```python
from build123d import *

# Parameters (mm, degrees)
F0_W     = 69.5
F0_H     = 23
F0_R     = 5.75
F0_W_2   = 1
F0_H_2   = 4
F1_DEPTH = 2
F0_R_2   = 5.25
F2_DEPTH = 10


with BuildPart() as f1:
    # F0 (on Top) → F1 (new body)
    with BuildSketch(Plane.XY):
        with Locations((3.4471642077, -3.0003356891)):
            Rectangle(F0_W, F0_H)
        Polygon((-29.8028357923, -13.0003356891), (-29.8028357923, 6.9996643109), (-15.8028357923, 6.9996643109), (-14.8028357923, 6.9996643109), (-13.3028357923, 6.9996643109), (-12.3028357923, 6.9996643109), (1.6971642077, 6.9996643109), (2.6971642077, 6.9996643109), (4.1971642077, 6.9996643109), (5.1971642077, 6.9996643109), (19.1971642077, 6.9996643109), (20.1971642077, 6.9996643109), (21.6971642077, 6.9996643109), (22.6971642077, 6.9996643109), (36.6971642077, 6.9996643109), (36.6971642077, -13.0003356891), (22.6971642077, -13.0003356891), (21.6971642077, -13.0003356891), (20.1971642077, -13.0003356891), (19.1971642077, -13.0003356891), (5.1971642077, -13.0003356891), (5.1971642077, -9.0003356891), (4.1971642077, -9.0003356891), (4.1971642077, -13.0003356891), (2.6971642077, -13.0003356891), (1.6971642077, -13.0003356891), (-12.3028357923, -13.0003356891), (-13.3028357923, -13.0003356891), (-14.8028357923, -13.0003356891), (-15.8028357923, -13.0003356891), align=None, mode=Mode.SUBTRACT)
        Polygon((-15.8028357923, 6.9996643109), (-29.8028357923, 6.9996643109), (-29.8028357923, -13.0003356891), (-15.8028357923, -13.0003356891), (-15.8028357923, -9.0003356891), (-14.8028357923, -9.0003356891), (-14.8028357923, -13.0003356891), (-13.3028357923, -13.0003356891), (-13.3028357923, -9.0003356891), (-12.3028357923, -9.0003356891), (-12.3028357923, -13.0003356891), (1.6971642077, -13.0003356891), (1.6971642077, -9.0003356891), (2.6971642077, -9.0003356891), (2.6971642077, -13.0003356891), (4.1971642077, -13.0003356891), (4.1971642077, -9.0003356891), (5.1971642077, -9.0003356891), (5.1971642077, -13.0003356891), (19.1971642077, -13.0003356891), (19.1971642077, -9.0003356891), (20.1971642077, -9.0003356891), (20.1971642077, -13.0003356891), (21.6971642077, -13.0003356891), (21.6971642077, -9.0003356891), (22.6971642077, -9.0003356891), (22.6971642077, -13.0003356891), (36.6971642077, -13.0003356891), (36.6971642077, 6.9996643109), (22.6971642077, 6.9996643109), (22.6971642077, 2.9996643109), (21.6971642077, 2.9996643109), (21.6971642077, 6.9996643109), (20.1971642077, 6.9996643109), (20.1971642077, 2.9996643109), (19.1971642077, 2.9996643109), (19.1971642077, 6.9996643109), (5.1971642077, 6.9996643109), (5.1971642077, 2.9996643109), (4.1971642077, 2.9996643109), (4.1971642077, 6.9996643109), (2.6971642077, 6.9996643109), (2.6971642077, 2.9996643109), (1.6971642077, 2.9996643109), (1.6971642077, 6.9996643109), (-12.3028357923, 6.9996643109), (-12.3028357923, 2.9996643109), (-13.3028357923, 2.9996643109), (-13.3028357923, 6.9996643109), (-14.8028357923, 6.9996643109), (-14.8028357923, 2.9996643109), (-15.8028357923, 2.9996643109), align=None)
        with Locations((-22.8028357923, -3.0003356891)):
            Circle(F0_R, mode=Mode.SUBTRACT)
        with Locations((-5.3028357923, -3.0003356891)):
            Circle(F0_R, mode=Mode.SUBTRACT)
        with Locations((12.1971642077, -3.0003356891)):
            Circle(F0_R, mode=Mode.SUBTRACT)
        with Locations((29.6971642077, -3.0003356891)):
            Circle(F0_R, mode=Mode.SUBTRACT)
        with Locations((-15.3028357923, 4.9996643109)):
            Rectangle(F0_W_2, F0_H_2)
        with Locations((-12.8028357923, 4.9996643109)):
            Rectangle(F0_W_2, F0_H_2)
        with Locations((2.1971642077, 4.9996643109)):
            Rectangle(F0_W_2, F0_H_2)
        with Locations((4.6971642077, 4.9996643109)):
            Rectangle(F0_W_2, F0_H_2)
        with Locations((19.6971642077, 4.9996643109)):
            Rectangle(F0_W_2, F0_H_2)
        with Locations((22.1971642077, 4.9996643109)):
            Rectangle(F0_W_2, F0_H_2)
        with Locations((-15.3028357923, -11.0003356891)):
            Rectangle(F0_W_2, F0_H_2)
        with Locations((-12.8028357923, -11.0003356891)):
            Rectangle(F0_W_2, F0_H_2)
        with Locations((2.1971642077, -11.0003356891)):
            Rectangle(F0_W_2, F0_H_2)
        with Locations((19.6971642077, -11.0003356891)):
            Rectangle(F0_W_2, F0_H_2)
        with Locations((22.1971642077, -11.0003356891)):
            Rectangle(F0_W_2, F0_H_2)
    extrude(amount=F1_DEPTH)

    # F0 (on Top) → F2 (join)
    with BuildSketch(Plane.XY):
        with Locations((-22.8028357923, -3.0003356891)):
            Circle(F0_R)
        with Locations((-22.8028357923, -3.0003356891)):
            Circle(F0_R_2, mode=Mode.SUBTRACT)
        with Locations((-5.3028357923, -3.0003356891)):
            Circle(F0_R)
        with Locations((-5.3028357923, -3.0003356891)):
            Circle(F0_R_2, mode=Mode.SUBTRACT)
        with Locations((12.1971642077, -3.0003356891)):
            Circle(F0_R)
        with Locations((12.1971642077, -3.0003356891)):
            Circle(F0_R_2, mode=Mode.SUBTRACT)
        with Locations((29.6971642077, -3.0003356891)):
            Circle(F0_R)
        with Locations((29.6971642077, -3.0003356891)):
            Circle(F0_R_2, mode=Mode.SUBTRACT)
    extrude(amount=F2_DEPTH)


solid = f1.part
```
Could you check a few things on this model? Use its own coordinates, in mm. A direction names the side the tool comes from. Coordinates: 2 decimals unless noted, no trailing zeros. Write each loop counter-clockwise with the first axis right and the second up, starting at its lowest first coordinate (ties: lowest second). Pieces come first, ordered by that corner, then holes. Notation, with made-up numbers: (59.5, -4.5) -> (84.5, -4.5) arc R32 cw to (84.5, 30.5) -> close; hole circle Ø9 at (84.5, -22). An arc over 180 degrees is marked (long way). One line per question, with ' | ' between items. Start each with the question number.
1. Please list where these lines run through material, in increasing order: line 1 along X through (y, z) = (-5.75, 1.25); line 2 along Z through (x, y) = (22, -2.75); line 3 along Y through (x, z) = (25, 6).
2. Will these pins go through, and if not, where does the flat tip stop? P1, Ø1, axis at x = -8.5, z = 5, coming from the +Y side; P2, Ø10, axis at x = 22.5, y = 0, coming from the -Z side; P3, Ø4, axis at x = -22, z = 6, coming from the -Y side.
3. For faces 4 (the face through (-31.303, -3, 1)), 5 (the face through (23.953, -2.748, 5.944)), which set-ups out of +Z, -Z, +X, -X, +Y, -Y let a thin tool reach every point of the face, with its end or its side?
4. If we section it at B-B (x = 26): Please give me the cut outline in (y, z).
5. If we section it at A-A (z = 3): Please give me the cut outline in (x, y).
6. If we section it at D-D (x = -14): Please give me the cut outline in (y, z).
7. Thinking about a two-plate mould opening in Y: for faces 1 (the face through (3, -14.5, 1)), 2 (the face through (-0.295, -1.423, 4.93)), 3 (the face through (10, -8, 10)), which applies, pulls with the +Y half, pulls with the -Y half, needs draft (parallel to the pull), parting line crosses it, or undercut?
8. If we section it at C-C (y = 0.5): Count the separate pieces of the cut face and the enclosed holes in it, and give its area (3 significant figures).
Return value:
1) line 1: x = -31.3 to -27.28, -18.33 to -9.78, -0.83 to 7.72, 16.67 to 25.22, 34.17 to 38.2 | line 2: z = 0 to 2 | line 3: y = -6.32 to -5.35, -0.66 to 0.32
2) P1: stops at y = 2.08 | P2: stops at z = 0 | P3: stops at y = -8.75
3) face 4: +Z, -Z, -X, +Y, -Y | face 5: +Z
4) outline: (-14.5, 0) -> (-6.73, 0) -> (-6.73, 10) -> (-7.4, 10) -> (-7.4, 2) -> (-14.5, 2) -> close; (0.73, 0) -> (8.5, 0) -> (8.5, 2) -> (1.4, 2) -> (1.4, 10) -> (0.73, 10) -> close
5) outline: circle Ø11.5 at (-22.8, -3); circle Ø11.5 at (-5.3, -3); circle Ø11.5 at (12.2, -3); circle Ø11.5 at (29.7, -3); hole circle Ø10.5 at (-22.8, -3); hole circle Ø10.5 at (-5.3, -3); hole circle Ø10.5 at (12.2, -3); hole circle Ø10.5 at (29.7, -3)
6) outline: (-14.5, 0) -> (8.5, 0) -> (8.5, 2) -> (-14.5, 2) -> close
7) face 1: pulls with the -Y half | face 2: undercut | face 3: needs draft
8) separate pieces: 5 | enclosed holes: 0 | area: 118 mm²
